Autodesk Inventor part; units mm, degrees
ref_plane "YZ Plane" through (0, 0, 0) normal (1, 0, 0) x (0, 1, 0)
ref_plane "XZ Plane" through (0, 0, 0) normal (0, 1, 0) x (-1, 0, 0)
ref_plane "XY Plane" through (0, 0, 0) normal (0, 0, 1) x (1, 0, 0)
sketch "Sketch1" plane through (0, 0, 0) normal (0, 0, 1) x (1, 0, 0)
  circle A0 centre (0, 0) radius 8
  dimension "d0" = 16
extrude "Extrusion1" add sketch "Sketch1" against normal blind 4
sketch "Sketch2" plane through (0, 0, -4) normal (0, 0, -1) x (-1, 0, 0)
  circle A0 centre (0, 0) radius 6
  dimension "d3" = 12
extrude "Extrusion2" add sketch "Sketch2" along normal blind 5.4
sketch "Sketch3" plane through (0, 0, -9.4) normal (0, 0, -1) x (-1, 0, 0)
  circle A0 centre (0, 0) radius 8
  circle A1 centre (0, 0) radius 8
extrude "Extrusion3" add sketch "Sketch3" along normal blind 3
sketch "Sketch4" plane through (0, 0, -12.4) normal (0, 0, -1) x (-1, 0, 0)
  circle A0 centre (0, 0) radius 4.7
  dimension "d8" = 9.4
extrude "Extrusion4" add sketch "Sketch4" along normal blind 4.32
sketch "Sketch5" plane through (0, 0, -16.72) normal (0, 0, -1) x (-1, 0, 0)
  circle A0 centre (0, 0) radius 11.25
  dimension "d11" = 22.5
extrude "Extrusion5" add sketch "Sketch5" along normal blind 1.35
sketch "Sketch6" plane through (0, 0, -18.07) normal (0, 0, -1) x (-1, 0, 0)
  circle A0 centre (0, 0) radius 4.7
extrude "Extrusion6" add sketch "Sketch6" along normal blind 2
sketch "Sketch7" plane through (0, 0, -20.07) normal (0, 0, -1) x (-1, 0, 0)
  circle A0 centre (0, 0) radius 11.25
  circle A1 centre (0, 0) radius 11.25
extrude "Extrusion7" add sketch "Sketch7" along normal blind 1.35
sketch "Sketch8" plane through (0, 0, -21.42) normal (0, 0, -1) x (-1, 0, 0)
  circle A0 centre (0, 0) radius 4.7
extrude "Extrusion8" add sketch "Sketch8" along normal blind 2
sketch "Sketch9" plane through (0, 0, -23.42) normal (0, 0, -1) x (-1, 0, 0)
  circle A0 centre (0, 0) radius 11.25
  circle A1 centre (0, 0) radius 11.25
extrude "Extrusion9" add sketch "Sketch9" along normal blind 1.35
sketch "Sketch10" plane through (0, 0, -24.77) normal (0, 0, -1) x (-1, 0, 0)
  circle A0 centre (0, 0) radius 4.7
extrude "Extrusion10" add sketch "Sketch10" along normal blind 2
sketch "Sketch11" plane through (0, 0, -26.77) normal (0, 0, -1) x (-1, 0, 0)
  circle A0 centre (0, 0) radius 11.25
  circle A1 centre (0, 0) radius 11.25
extrude "Extrusion11" add sketch "Sketch11" along normal blind 1.35
sketch "Sketch12" plane through (0, 0, -28.12) normal (0, 0, -1) x (-1, 0, 0)
  circle A0 centre (0, 0) radius 4.7
extrude "Extrusion12" add sketch "Sketch12" along normal blind 2
sketch "Sketch13" plane through (0, 0, -30.12) normal (0, 0, -1) x (-1, 0, 0)
  circle A0 centre (0, 0) radius 11.25
  circle A1 centre (0, 0) radius 11.25
extrude "Extrusion13" add sketch "Sketch13" along normal blind 1.35
sketch "Sketch14" plane through (0, 0, -31.47) normal (0, 0, -1) x (-1, 0, 0)
  circle A0 centre (0, 0) radius 4.7
extrude "Extrusion14" add sketch "Sketch14" along normal blind 2
sketch "Sketch15" plane through (0, 0, -33.47) normal (0, 0, -1) x (-1, 0, 0)
  circle A0 centre (0, 0) radius 11.25
  circle A1 centre (0, 0) radius 11.25
extrude "Extrusion15" add sketch "Sketch15" along normal blind 1.35
sketch "Sketch16" plane through (0, 0, -34.82) normal (0, 0, -1) x (-1, 0, 0)
  circle A0 centre (0, 0) radius 4.7
extrude "Extrusion16" add sketch "Sketch16" along normal blind 2
sketch "Sketch17" plane through (0, 0, -36.82) normal (0, 0, -1) x (-1, 0, 0)
  circle A0 centre (0, 0) radius 11.25
  circle A1 centre (0, 0) radius 11.25
extrude "Extrusion17" add sketch "Sketch17" along normal blind 1.35
sketch "Sketch18" plane through (0, 0, -38.17) normal (0, 0, -1) x (-1, 0, 0)
  circle A0 centre (0, 0) radius 4.7
extrude "Extrusion18" add sketch "Sketch18" along normal blind 2
sketch "Sketch19" plane through (0, 0, -40.17) normal (0, 0, -1) x (-1, 0, 0)
  circle A0 centre (0, 0) radius 11.25
  circle A1 centre (0, 0) radius 11.25
extrude "Extrusion19" add sketch "Sketch19" along normal blind 1.35
sketch "Sketch20" plane through (0, 0, -41.52) normal (0, 0, -1) x (-1, 0, 0)
  circle A0 centre (0, 0) radius 4.7
extrude "Extrusion20" add sketch "Sketch20" along normal blind 2
sketch "Sketch21" plane through (0, 0, -43.52) normal (0, 0, -1) x (-1, 0, 0)
  circle A0 centre (0, 0) radius 11.25
  circle A1 centre (0, 0) radius 11.25
extrude "Extrusion21" add sketch "Sketch21" along normal blind 1.35
sketch "Sketch22" plane through (0, 0, -44.87) normal (0, 0, -1) x (-1, 0, 0)
  circle A0 centre (0, 0) radius 4.7
extrude "Extrusion22" add sketch "Sketch22" along normal blind 2
sketch "Sketch23" plane through (0, 0, -46.87) normal (0, 0, -1) x (-1, 0, 0)
  circle A0 centre (0, 0) radius 11.25
  circle A1 centre (0, 0) radius 11.25
extrude "Extrusion23" add sketch "Sketch23" along normal blind 1.35
sketch "Sketch24" plane through (0, 0, -48.22) normal (0, 0, -1) x (-1, 0, 0)
  circle A0 centre (0, 0) radius 3
  dimension "d50" = 6
extrude "Extrusion24" add sketch "Sketch24" along normal blind 3.6
sketch "Sketch25" plane through (0, 0, -51.82) normal (0, 0, -1) x (-1, 0, 0)
  line L0 (5.25, -8.25) -> (-11.25, -8.25)
  line L1 (-11.25, -8.25) -> (-11.25, 8.25)
  line L2 (-11.25, 8.25) -> (5.25, 8.25)
  line L3 (5.25, 8.25) -> (5.25, -8.25)
  circle A0 centre (0, 0) radius 11.25
  point P0 (5.25, 0)
  dimension "d53" = 16.5
  dimension "d54" = 16.5
extrude "Extrusion25" add sketch "Sketch25" along normal blind 11.5 contours L0 A0 L2 L3 | L0 L1 A0 | L1 L2 A0 picked at (-0.25, 0)
sketch "Sketch26" plane through (0, 0, -63.32) normal (0, 0, -1) x (-1, 0, 0)
  circle A0 centre (0, 0) radius 3
  line L0 (-4, -2.3094) -> (-4, 2.3094)
  line L1 (-4, 2.3094) -> (0, 4.6188)
  line L2 (0, 4.6188) -> (4, 2.3094)
  line L3 (4, 2.3094) -> (4, -2.3094)
  line L4 (4, -2.3094) -> (0, -4.6188)
  line L5 (0, -4.6188) -> (-4, -2.3094)
  line L6 (5.25, -8.25) -> (5.25, 8.25)
  dimension "d58" = 8
extrude "Extrusion26" add sketch "Sketch26" along normal blind 5 contours A0 | L0 L1 L2 L3 L4 L5
chamfer "Chamfer1" distance 3.7 angle 45 6 edges at (-4, 0, -68.32) (-2, 3.4641, -68.32) (2, 3.4641, -68.32) (4, 0, -68.32) (2, -3.4641, -68.32) (-2, -3.4641, -68.32)
sketch "Sketch27" plane through (0, 0, -68.32) normal (0, 0, -1) x (-1, 0, 0)
  circle A0 centre (0, 0) radius 0.2
  dimension "d64" = 0.4
extrude "Extrusion27" cut sketch "Sketch27" against normal blind 75.75
sketch "Sketch28" plane through (0, 0, 0) normal (0, 0, 1) x (1, 0, 0)
  circle A0 centre (0, 0) radius 1
  dimension "d67" = 2
extrude "Extrusion28" cut sketch "Sketch28" against normal blind 61.5
sketch "Sketch29" plane through (0, 0, 0) normal (0, 0, 1) x (1, 0, 0)
  circle A0 centre (0, 0) radius 0.2
  circle A1 centre (0, 0) radius 4.75
  dimension "d70" = 9.5
extrude "Extrusion29" cut sketch "Sketch29" against normal blind 8 contours A0 | A1
chamfer "Chamfer2" distance 3.75 angle 45 1 edges at (-1, 0, -8)
thread "Thread1"
chamfer "Chamfer3" distance 0.2 angle 45 25 edges at (-8, 0, 0) (-8, 0, -4) (8, 0, -9.4) (8, 0, -12.4) (-4.75, 0, 0) (11.25, 0, -16.72) (11.25, 0, -18.07) (11.25, 0, -20.07) (11.25, 0, -21.42) (11.25, 0, -23.42) (11.25, 0, -24.77) (11.25, 0, -26.77) (11.25, 0, -28.12) (11.25, 0, -30.12) (11.25, 0, -31.47) (11.25, 0, -33.47) (11.25, 0, -34.82) (11.25, 0, -36.82) (11.25, 0, -38.17) (11.25, 0, -40.17) (11.25, 0, -41.52) (11.25, 0, -43.52) (11.25, 0, -44.87) (11.25, 0, -46.87) (11.25, 0, -48.22)
chamfer "Chamfer4" distance 0.2 angle 45 4 edges at (-5.25, -8.25, -57.57) (11.25, -8.25, -57.57) (-5.25, 8.25, -57.57) (11.25, 8.25, -57.57)
thread "Thread2"
sketch "Sketch30" plane through (-5.05, 8.25, -51.82) normal (0, 1, 0) x (1, 0, 0)
  circle A0 centre (11.8, 6.0984) radius 3
  line L0 (16.3, 0) -> (16.3, 11.5)
  point P0 (5.05, -51.82)
  dimension "d86" = 6
  dimension "d87" = 4.5
extrude "Extrusion30" cut sketch "Sketch30" against normal blind 16.5
chamfer "Chamfer5" distance 0.2 angle 45 2 edges at (3.75, -8.25, -57.9184) (3.75, 8.25, -57.9184)
chamfer "Chamfer6" distance 0.2 angle 45 16 edges at (3, -8.25, -51.82) (11.25, 0, -51.82) (3, 8.25, -51.82) (-5.25, 0, -51.82) (-5.15, -8.15, -51.82) (11.15, -8.15, -51.82) (11.15, 8.15, -51.82) (-5.15, 8.15, -51.82) (-5.15, 8.15, -63.32) (-5.15, -8.15, -63.32) (11.15, -8.15, -63.32) (11.15, 8.15, -63.32) (3, 8.25, -63.32) (11.25, 0, -63.32) (3, -8.25, -63.32) (-5.25, 0, -63.32)
properties part number "Extruder Heat Sink" material "Aluminum 6061-AHC"
Geometry check sheet. Reference: the model listing, model coordinates, mm. A direction names the side the tool comes from. Coordinates: 2 decimals unless noted, no trailing zeros. Loops run counter-clockwise (first coordinate to the right, second up) from the corner with the lowest first, then second, coordinate; pieces in that order, holes last. Notation, with made-up numbers: (29, 67.25) - (66, 67.25) arc R21 ccw to (66, 103.25) - close; hole circle Ø8 at (78.5, -26). An arc over 180 degrees is marked (long way). Use one line per item in the form item = value. Start each with the question number.
Item 1: Thickness scan on probe 1 along Y at (x, z) = (0, -26.5); probe 2 along Y at (x, z) = (0, -64); probe 3 along Z at (x, y) = (9.5, 6.75). Record the ranges inside material, lowest first.
Item 2: Section check B-B, the plane z = -57. Give the number of separate pieces and of enclosed holes in the cut face, and give its area (3 significant figures).
Item 3: Tool access check on faces 5 (the face through (0, -5, -31.47)), 6 (the face through (8.36, 0.11, -60.45)), 7 (the face through (-5.19, 9.98, -44.19)). Record the directions out of +Z, -Z, +X, -X, +Y, -Y that give a thin tool (end or side, any length) a straight path to the whole face; none if there is none.
Item 4: Gauge pin test, flat ends, axial feed: pin 1 (8 mm diameter, centred on x = -4.5, y = 7.5, fed in from +Z); pin 2 (2 mm diameter, centred on x = -3, z = -15.5, fed in from +Y); pin 3 (12 mm diameter, centred on x = 8, z = -34, fed in from +Y); pin 4 (7 mm diameter, centred on x = 6.75, z = -57.92, fed in from +Y). Record the tip position at first contact, or that the pin passes through.
Item 5: Mould release check, pull along X, two halves, no side actions. Record for faces 1 (the face through (-5.19, 9.98, -34.14)), 2 (the face through (0, -1, -36)), 3 (the face through (-1.97, 3.48, -63.96)), 4 (the face through (0, -5, -33.47)): +X half, -X half, draft (parallel to the pull), parting line (faces both ways), or undercut.
Item 6: Section check A-A, the plane z = -39.5. Enter the section's corners in (x, y).
Computed:
q1.probe_1 = -4.7 to -1, 1 to 4.7
q1.probe_2 = -4.62 to -0.2, 0.2 to 4.62
q1.probe_3 = -63.32 to -59.12, -56.72 to -51.82
q2.separate_pieces = 2
q2.enclosed_holes = 1
q2.area = 175 mm2
q3.face_5 = none
q3.face_6 = +Y, -Y
q3.face_7 = +Z
q4.pin_1 = 0
q4.pin_2 = 4.25
q4.pin_3 = 11.07
q4.pin_4 = 8.25
q5.face_1 = parting line
q5.face_2 = undercut
q5.face_3 = -X half
q5.face_4 = draft
q6.outline = circle Ø9.4 at (0, 0); hole circle Ø2 at (0, 0)
